Geometry check sheet. Reference: the model listing, model coordinates, mm. A direction names the side the tool comes from. Give positions to 0.01 mm unless a question says otherwise; leave off trailing zeros. Write each loop counter-clockwise with the first axis right and the second up, starting at its lowest first coordinate (ties: lowest second). Pieces come first, ordered by that corner, then holes.
(1) Thickness scan on line 1 along X through (y, z) = (0.5, 276.5); line 2 along Y through (x, z) = (44.5, 257) (3 decimals); line 3 along Y through (x, z) = (-41.5, 269) (3 decimals). Record the ranges inside material, lowest first.
(2) Depth check by flat-ended pin: P1, Ø4, axis at x = 15.5, z = 146.5, coming from the -Y side (3 decimals); P2, Ø5, axis at x = 48.5, z = 56, coming from the -Y side (3 decimals); P3, Ø8, axis at y = -54, z = 16.5, coming from the -X side. Enter the tip coordinate at first touch or a pass-through.
(3) Cross-section at D-D (z = 215.5). Record the boundary of the cut face in (x, y) (3 decimals).
(4) Tool access check on faces 1 (the flat face through (19, 17.145, 5)), 2 (the flat face through (-44.45, -3, 5)), 3 (the flat face through (0, -122.555, 0)). Record the directions out of +Z, -Z, +X, -X, +Y, -Y that give a thin tool (end or side, any length) a straight path to the whole face; none if there is none.
(5) Cross-section at B-B (x = 0). Record the boundary of the cut face in (y, z) (3 decimals).
(6) Mould release check, pull along X, two halves, no side actions. Record for faces 4 (the flat face through (-50.8, 0, 5)), 5 (the flat face through (50.8, 0, 5)), 6 (the flat face through (1, 23.495, 5)), 7 (the cylindrical face through (-15.12, -51.73, -11.59)): +X half, -X half, draft (parallel to the pull), parting line (faces both ways), or undercut.
(7) Cross-section at C-C (z = 0). Record the boundary of the cut face in (x, y) (3 decimals).
(8) Cross-section at A-A (y = 7.5). Record the boundary of the cut face in (x, z), and give its area (3 significant figures).
```python
from build123d import *

# Parameters (mm, degrees)
BOSS_EXTRUDE1_DEPTH = 330.2
SKETCH2_R           = 19.05
BOSS_EXTRUDE2_DEPTH = 139.7


with BuildPart() as part:
    # Sketch1 → Boss-Extrude1 (new body, symmetric)
    with BuildSketch(Plane.XY):
        Polygon((-50.8, -23.495), (-44.45, -23.495), (-44.45, 17.145), (44.45, 17.145), (44.45, -23.495), (50.8, -23.495), (50.8, 23.495), (-50.8, 23.495), align=None)
    extrude(amount=BOSS_EXTRUDE1_DEPTH, both=True)

    # Sketch2 → Boss-Extrude2 (add)
    with BuildSketch(Plane.XZ.offset(-17.145)):
        Circle(SKETCH2_R)
    extrude(amount=BOSS_EXTRUDE2_DEPTH)


solid = part.part
```
Reply:
1. line 1: x = -50.8 to -44.45, 44.45 to 50.8
1. line 2: y = -23.495 to 23.495
1. line 3: y = 17.145 to 23.495
2. P1: stops at y = 17.145
2. P2: stops at y = -23.495
2. P3: stops at x = -14.38
3. outline: (-50.8, -23.495) - (-44.45, -23.495) - (-44.45, 17.145) - (44.45, 17.145) - (44.45, -23.495) - (50.8, -23.495) - (50.8, 23.495) - (-50.8, 23.495) - close
4. face 1: -Y
4. face 2: +Z, -Z, -Y
4. face 3: +Z, -Z, +X, -X, -Y
5. outline: (-122.555, -19.05) - (17.145, -19.05) - (17.145, -330.2) - (23.495, -330.2) - (23.495, 330.2) - (17.145, 330.2) - (17.145, 19.05) - (-122.555, 19.05) - close
6. face 4: -X half
6. face 5: +X half
6. face 6: draft
6. face 7: undercut
7. outline: (-50.8, -23.495) - (-44.45, -23.495) - (-44.45, 17.145) - (-19.05, 17.145) - (-19.05, -122.555) - (19.05, -122.555) - (19.05, 17.145) - (44.45, 17.145) - (44.45, -23.495) - (50.8, -23.495) - (50.8, 23.495) - (-50.8, 23.495) - close
8. outline: (-50.8, -330.2) - (-44.45, -330.2) - (-44.45, 330.2) - (-50.8, 330.2) - close; circle Ø38.1 at (0, 0); (44.45, -330.2) - (50.8, -330.2) - (50.8, 330.2) - (44.45, 330.2) - close
8. area: 9,530 mm2
